```python
from build123d import *

# Parameters (mm, degrees)
ESQUISSE1_W                       = 30
ESQUISSE1_H                       = 30
BASE_EXTRUSION_DEPTH              = 12
ESQUISSE2_R                       = 12
ESQUISSE2_R_2                     = 10
BOS_EXTRU_MINCE1_DEPTH            = 25
ESQUISSE3_W                       = 30
ESQUISSE3_H                       = 30
BOSS_EXTRU_1_DEPTH                = 12
BOSS_EXTRU_2_REACH                = 58.294
ESQUISSE4_R                       = 2
BOSS_EXTRU_3_REACH                = 53.124
ESQUISSE5_R                       = 2
BOSS_EXTRU_4_REACH                = 64.884
ESQUISSE6_R                       = 2
BOSS_EXTRU_5_REACH                = 69.61
ESQUISSE7_R                       = 2
ESQUISSE10_R                      = 9
BOSS_EXTRU_6_DEPTH                = 6
EXTRUSION1_START                  = 13
ESQUISSE15_R                      = 2
EXTRUSION1_DEPTH                  = 13
ESQUISSE16_R                      = 2
EXTRUSION2_DEPTH                  = 5
CHANFREIN2_SIZE                   = 0.5
CHANFREIN5_SIZE                   = 1
ESQUISSE17_R                      = 4
ENL_V_MAT_EXTRU_1_DEPTH           = 26.67049611
CHANFREIN6_SIZE                   = 2
ESQUISSE24_R                      = 7.5
ESQUISSE24_R_2                    = 6.5
ENL_V_MAT_EXTRU_2_DEPTH           = 8
ESQUISSE25_R                      = 6.5
ENL_V_MAT_EXTRU_3_DEPTH           = 4
CHANFREIN7_SIZE                   = 1
DIAM_TRE_DU_PER_AGE_4_0_4_1_D     = 4
DIAM_TRE_DU_PER_AGE_4_0_4_1_DEPTH = 17
DIAM_TRE_DU_PER_AGE_4_0_4_1_TIP   = 1.201721238
ESQUISSE28_R                      = 2
ENL_V_MAT_EXTRU_4_DEPTH           = 5


with BuildPart() as part:
    # Esquisse1 → Base-Extrusion (new body)
    with BuildSketch(Plane.XY):
        with Locations((15, 15)):
            Rectangle(ESQUISSE1_W, ESQUISSE1_H)
    extrude(amount=BASE_EXTRUSION_DEPTH)

    # Esquisse2 → Bos.-Extru.-Mince1 (add)
    with BuildSketch(Plane.XY.offset(12)):
        with Locations((15, 15)):
            Circle(ESQUISSE2_R)
        with Locations((15, 15)):
            Circle(ESQUISSE2_R_2, mode=Mode.SUBTRACT)
    extrude(amount=BOS_EXTRU_MINCE1_DEPTH)

    # Esquisse3 → Boss.-Extru.1 (add)
    with BuildSketch(Plane.XY.offset(37)):
        with Locations((15, 15)):
            Rectangle(ESQUISSE3_W, ESQUISSE3_H)
    extrude(amount=BOSS_EXTRU_1_DEPTH)

    # Esquisse4 → Boss.-Extru.2 (add, up to next)
    with BuildSketch(Plane.XY.offset(12), mode=Mode.PRIVATE) as boss_extru_2_sk1:
        with Locations(Location((4, 26, 0), (0, 0, 180))):
            Circle(ESQUISSE4_R)
    boss_extru_2_tool1 = extrude(boss_extru_2_sk1.sketch, amount=BOSS_EXTRU_2_REACH, mode=Mode.PRIVATE) - part.part
    add(boss_extru_2_tool1.solids().sort_by_distance((4, 26, 12))[0])

    # Esquisse5 → Boss.-Extru.3 (add, up to next)
    with BuildSketch(Plane(origin=(19.916830052, 0.880144556, 12), x_dir=(1, 0, 0), z_dir=(0, 0, 1)), mode=Mode.PRIVATE) as boss_extru_3_sk1:
        with Locations(Location((6.083169948, 25.119855444, 0), (0, 0, 180))):
            Circle(ESQUISSE5_R)
    boss_extru_3_tool1 = extrude(boss_extru_3_sk1.sketch, amount=BOSS_EXTRU_3_REACH, mode=Mode.PRIVATE) - part.part
    add(boss_extru_3_tool1.solids().sort_by_distance((26, 26, 12))[0])

    # Esquisse6 → Boss.-Extru.4 (add, up to next)
    with BuildSketch(Plane(origin=(19.426828301, -16.989020523, 12), x_dir=(1, 0, 0), z_dir=(0, 0, 1)), mode=Mode.PRIVATE) as boss_extru_4_sk1:
        with Locations(Location((6.573171699, 20.989020523, 0), (0, 0, 180))):
            Circle(ESQUISSE6_R)
    boss_extru_4_tool1 = extrude(boss_extru_4_sk1.sketch, amount=BOSS_EXTRU_4_REACH, mode=Mode.PRIVATE) - part.part
    add(boss_extru_4_tool1.solids().sort_by_distance((26, 4, 12))[0])

    # Esquisse7 → Boss.-Extru.5 (add, up to next)
    with BuildSketch(Plane(origin=(0.731824689, -18.430102912, 12), x_dir=(1, 0, 0), z_dir=(0, 0, 1)), mode=Mode.PRIVATE) as boss_extru_5_sk1:
        with Locations(Location((3.268175311, 22.430102912, 0), (0, 0, 180))):
            Circle(ESQUISSE7_R)
    boss_extru_5_tool1 = extrude(boss_extru_5_sk1.sketch, amount=BOSS_EXTRU_5_REACH, mode=Mode.PRIVATE) - part.part
    add(boss_extru_5_tool1.solids().sort_by_distance((4, 4, 12))[0])

    # Esquisse10 → Boss.-Extru.6 (add)
    with BuildSketch(Plane(origin=(0, 0, 0), x_dir=(-1, 0, 0), z_dir=(0, 0, -1))):
        with Locations(Location((-15, 15, 0), (0, 0, 180))):
            Circle(ESQUISSE10_R)
    extrude(amount=BOSS_EXTRU_6_DEPTH)

    # Esquisse15 → Extrusion1 (add)
    with BuildSketch(Plane(origin=(0, 0, 0), x_dir=(-1, 0, 0), z_dir=(0, 0, -1)).offset(EXTRUSION1_START)):
        with Locations((-4, 26)):
            Circle(ESQUISSE15_R)
        with Locations((-4, 4)):
            Circle(ESQUISSE15_R)
        with Locations((-26, 4)):
            Circle(ESQUISSE15_R)
        with Locations((-26, 26)):
            Circle(ESQUISSE15_R)
    extrude(amount=-EXTRUSION1_DEPTH)

    # Esquisse16 → Extrusion2 (add)
    with BuildSketch(Plane.XY.offset(49)):
        with Locations(Location((26, 26, 0), (0, 0, 180))):
            Circle(ESQUISSE16_R)
        with Locations(Location((26, 4, 0), (0, 0, 180))):
            Circle(ESQUISSE16_R)
        with Locations(Location((4, 4, 0), (0, 0, 180))):
            Circle(ESQUISSE16_R)
        with Locations(Location((4, 26, 0), (0, 0, 180))):
            Circle(ESQUISSE16_R)
    extrude(amount=EXTRUSION2_DEPTH)

    # Chanfrein2
    chanfrein2_edges = [part.edges().sort_by_distance(p)[0] for p in [
        (6, 26, -13),
        (6, 4, -13),
        (28, 4, -13),
        (28, 26, -13),
        (28, 26, 54),
        (28, 4, 54),
        (6, 4, 54),
        (6, 26, 54),
    ]]
    chamfer(chanfrein2_edges, length=CHANFREIN2_SIZE)

    # Chanfrein5
    chanfrein5_edges = [part.edges().sort_by_distance(p)[0] for p in [
        (6, 15, -6),
    ]]
    chamfer(chanfrein5_edges, length=CHANFREIN5_SIZE)

    # Esquisse17 → Enlèv. mat.-Extru.1 (cut)
    with BuildSketch(Plane(origin=(0, 0, -6), x_dir=(-1, 0, 0), z_dir=(0, 0, -1))):
        with Locations((-15, 15)):
            Circle(ESQUISSE17_R)
    extrude(amount=-ENL_V_MAT_EXTRU_1_DEPTH, mode=Mode.SUBTRACT)

    # Chanfrein6
    chanfrein6_edges = [part.edges().sort_by_distance(p)[0] for p in [
        (0, 30, 43),
        (0, 0, 43),
        (30, 0, 43),
        (30, 30, 43),
        (0, 30, 6),
        (30, 30, 6),
        (30, 0, 6),
        (0, 0, 6),
    ]]
    chamfer(chanfrein6_edges, length=CHANFREIN6_SIZE)

    # Esquisse24 → Enlèv. mat.-Extru.2 (cut)
    with BuildSketch(Plane.XY.offset(12)):
        with Locations((15, 15)):
            Circle(ESQUISSE24_R)
        with Locations((15, 15)):
            Circle(ESQUISSE24_R_2, mode=Mode.SUBTRACT)
    extrude(amount=-ENL_V_MAT_EXTRU_2_DEPTH, mode=Mode.SUBTRACT)

    # Esquisse25 → Enlèv. mat.-Extru.3 (cut)
    with BuildSketch(Plane.XY.offset(12)):
        with Locations((15, 15)):
            Circle(ESQUISSE25_R)
    extrude(amount=-ENL_V_MAT_EXTRU_3_DEPTH, mode=Mode.SUBTRACT)

    # Chanfrein7
    chanfrein7_edges = [part.edges().sort_by_distance(p)[0] for p in [
        (8.5, 15, 8),
    ]]
    chamfer(chanfrein7_edges, length=CHANFREIN7_SIZE)

    # Diamètre du perçage Ø4.0 (4)1
    with Locations(Plane(origin=(0, 30, 0), x_dir=(-1, 0, 0), z_dir=(0, 1, 0))):
        with Locations((-15, 42)):
            Hole(DIAM_TRE_DU_PER_AGE_4_0_4_1_D / 2, depth=DIAM_TRE_DU_PER_AGE_4_0_4_1_DEPTH)
            with Locations((0, 0, -(DIAM_TRE_DU_PER_AGE_4_0_4_1_DEPTH + DIAM_TRE_DU_PER_AGE_4_0_4_1_TIP / 2))):  # 118° drill point
                Cone(0, DIAM_TRE_DU_PER_AGE_4_0_4_1_D / 2, DIAM_TRE_DU_PER_AGE_4_0_4_1_TIP, mode=Mode.SUBTRACT)

    # Esquisse28 → Enlèv. mat.-Extru.4 (cut)
    with BuildSketch(Plane(origin=(0, 0, 37), x_dir=(-1, 0, 0), z_dir=(0, 0, -1))):
        with Locations((-15, 15)):
            Circle(ESQUISSE28_R)
    extrude(amount=-ENL_V_MAT_EXTRU_4_DEPTH, mode=Mode.SUBTRACT)


solid = part.part
```
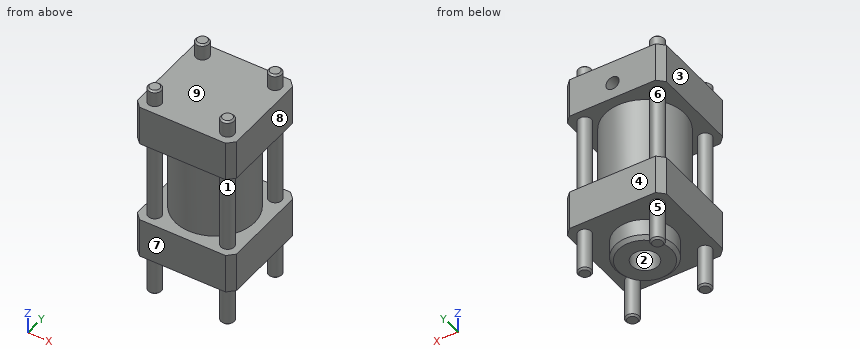
The listing builds one solid part. Answer for the finished solid, in the listing's coordinates (mm). Face numbers are marked on the shaded views. A direction names the side the tool comes from. Round coordinates to 2 decimals unless told otherwise and drop trailing zeros. Loops run counter-clockwise (first coordinate to the right, second up) from the corner with the lowest first, then second, coordinate; pieces in that order, holes last.
1) Consider line 1 (Y direction, x = 15, z = 18.25); line 2 (Z direction, x = 3.5, y = 20.25); line 3 (Z direction, x = 18.5, y = 21). Determine where each line is inside the solid, lowest interval first.
Outcome:
line 1: y = 3 to 5, 25 to 27
line 2: z = 0 to 12, 37 to 49
line 3: z = -6 to 4, 37 to 49
2) Given P1, Ø1, axis at x = 17.5, y = 14.5, coming from the +Z side; P2, Ø16, axis at x = 15, y = 15, coming from the -Z side; P3, Ø6, axis at x = 23.5, z = 13, coming from the -Y side; P4, Ø5, axis at x = 15, y = 15, coming from the -Z side, each flat-ended and moving along its own axis, determine where each tip first touches the part or whether it passes through.
Outcome:
P1: stops at z = 49
P2: stops at z = -6
P3: stops at y = 0
P4: stops at z = 37
3) A cutting plane is placed at B-B on x = 25.75. Give the number of separate pieces and of enclosed holes in the cut face, plus the area to 3 significant figures.
Outcome:
separate pieces: 1
enclosed holes: 2
area: 1,330 mm2
4) For a pull along Y with two mould halves and no side action, classify the marked faces 1, 2, 3 and 4 as released by +Y, released by -Y, zero draft, split by the parting line, or undercut.
Outcome:
face 1: undercut
face 2: undercut
face 3: zero draft
face 4: released by +Y
5) For the marked faces 5, 6, 7, 8 and 9, determine the directions among +Z, -Z, +X, -X, +Y, -Y from which every point of the face is accessible in a straight line to the end or side of a thin tool.
Outcome:
face 5: -Z
face 6: none
face 7: +Z, -Z, +X, -X, -Y
face 8: +Z, -Z, +X, +Y, -Y
face 9: +Z
6) A cutting plane is placed at A-A on z = 20. Determine the outline of the cut face in (x, y), plus the area to 3 significant figures.
Outcome:
outline: circle Ø4 at (4, 4); circle Ø4 at (4, 26); circle Ø24 at (15, 15); circle Ø4 at (26, 4); circle Ø4 at (26, 26); hole circle Ø20 at (15, 15)
area: 188 mm2
